CAD build for the part. Positions are in the model's coordinates, mm. Give positions to 0.01 mm unless a question says otherwise; leave off trailing zeros. Write each loop counter-clockwise with the first axis right and the second up, starting at its lowest first coordinate (ties: lowest second). Pieces come first, ordered by that corner, then holes. Notation, with made-up numbers: (-37, -17) - (-16, -17) arc R27 cw to (-16, 16) - close; hole circle Ø11 at (-29, 34.25). An arc over 180 degrees is marked (long way). Write item = value, one per line. Start each with the question number.
```python
from build123d import *

# Parameters (mm, degrees)
SKETCH1_W           = 50.8
SKETCH1_H           = 50.8
BOSS_EXTRUDE1_DEPTH = 5.08
SKETCH11_R          = 0.7366
BOSS_EXTRUDE2_DEPTH = 2.286
SKETCH12_W          = 45.72
SKETCH12_H          = 45.72
CUT_EXTRUDE1_DEPTH  = 1.27


with BuildPart() as part:
    # Sketch1 → Boss-Extrude1 (new body)
    with BuildSketch(Plane(origin=(0, 0, 0), x_dir=(1, 0, 0), z_dir=(0, 1, 0))):
        Rectangle(SKETCH1_W, SKETCH1_H)
    extrude(amount=BOSS_EXTRUDE1_DEPTH)

    # Sketch11 → Boss-Extrude2 (add)
    with BuildSketch(Plane(origin=(0, 5.08, 0), x_dir=(1, 0, 0), z_dir=(0, 1, 0))):
        with Locations(Location((-24.142764143, 24.142764143, 0), (0, 0, 90))):
            Circle(SKETCH11_R)
        with Locations(Location((24.142764143, 24.142764143, 0), (0, 0, 90))):
            Circle(SKETCH11_R)
        with Locations(Location((24.142764143, -24.142764143, 0), (0, 0, 90))):
            Circle(SKETCH11_R)
        with Locations(Location((-24.142764143, -24.142764143, 0), (0, 0, 90))):
            Circle(SKETCH11_R)
    extrude(amount=BOSS_EXTRUDE2_DEPTH)

    # Sketch12 → Cut-Extrude1 (cut)
    with BuildSketch(Plane.XZ):
        Rectangle(SKETCH12_W, SKETCH12_H)
    extrude(amount=-CUT_EXTRUDE1_DEPTH, mode=Mode.SUBTRACT)


solid = part.part
```
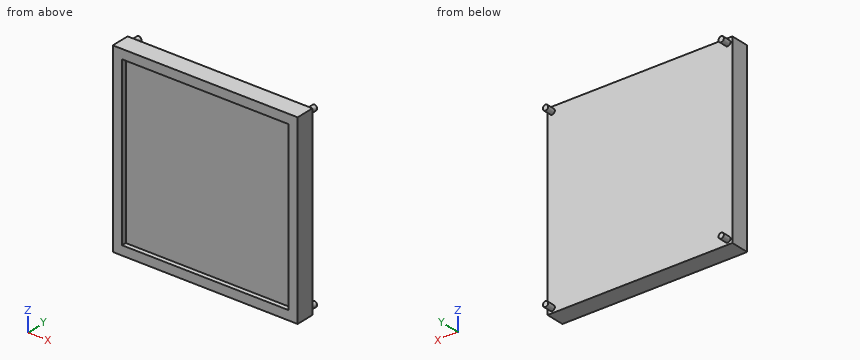
1. Wall check: line 1 along X through (y, z) = (1, -18); line 2 along Y through (x, z) = (0, -9.5). Give the ranges that are in metal, low to high.
2. Pin check, flat tips, straight feed: pin 1 Ø6 at (x, z) = (8, 4.5) entering from +Y; pin 2 Ø5 at (x, z) = (9.5, -9) entering from -Y. Stop position of each tip, or through.
3. Cut at B-B (x = -18.5). Give the cut face in (y, z), then the cut area to 3 significant figures.
4. Cut at A-A (z = -4.5). Give the cut face in (x, y), then the cut area to 3 significant figures.
Output:
q1.line_1 = -25.4 to -22.86, 22.86 to 25.4
q1.line_2 = 1.27 to 5.08
q2.pin_1 = 5.08
q2.pin_2 = 1.27
q3.outline = (0, -25.4) - (5.08, -25.4) - (5.08, 25.4) - (0, 25.4) - (0, 22.86) - (1.27, 22.86) - (1.27, -22.86) - (0, -22.86) - close
q3.area = 200 mm2
q4.outline = (-25.4, 0) - (-22.86, 0) - (-22.86, 1.27) - (22.86, 1.27) - (22.86, 0) - (25.4, 0) - (25.4, 5.08) - (-25.4, 5.08) - close
q4.area = 200 mm2
